Could you check a few things on this model? Use its own coordinates, in mm. A direction names the side the tool comes from. Coordinates: 2 decimals unless noted, no trailing zeros. Loops run counter-clockwise (first coordinate to the right, second up) from the corner with the lowest first, then second, coordinate; pieces in that order, holes last.
from build123d import *

# Parameters (mm, degrees)
SKETCH_R        = 6
SKETCH_R_2      = 4
PAD_DEPTH       = 8
PAD001_DEPTH    = 3
SKETCH002_W     = 2
SKETCH002_H     = 10
SKETCH002_W_2   = 10
SKETCH002_H_2   = 2
PAD002_DEPTH    = 2
CHAMFER_SIZE    = 1.99
CHAMFER001_SIZE = 1.99
PAD003_DEPTH    = 6
PAD003_FACE20_W = 5.5
PAD003_FACE20_H = 5.5
POCKET_DEPTH    = 11.001
FILLET_R        = 1
CHAMFER002_SIZE = 1.5


with BuildPart() as part:
    # Sketch → Pad (new body)
    with BuildSketch(Plane.XY):
        with Locations((15, 15)):
            Circle(SKETCH_R)
        with Locations((15, 15)):
            Circle(SKETCH_R_2, mode=Mode.SUBTRACT)
    extrude(amount=PAD_DEPTH)

    # Sketch001 (on Face4 of Pad) → Pad001 (join)
    with BuildSketch(Plane.XY.offset(8)):
        with BuildLine():
            Line((0, 28.183589), (0, 0))
            Line((0, 0), (28.371979, 0))
            ThreePointArc((28.371979, 0), (29.515053, 0.439592), (29.949498, 1.584632))
            ThreePointArc((29.949498, 1.584632), (21.158025, 21.174653), (1.561155, 29.950849))
            ThreePointArc((1.561155, 29.950849), (0.351368, 29.446372), (0, 28.183589))
        make_face()
    extrude(amount=PAD001_DEPTH)

    # Sketch002 (on Face4 of Pad001) → Pad002 (join)
    with BuildSketch(Plane(origin=(0, 0, 8), x_dir=(1, 0, 0), z_dir=(0, 0, -1))):
        with Locations((6, -15)):
            Rectangle(SKETCH002_W, SKETCH002_H)
        with Locations((15, -6)):
            Rectangle(SKETCH002_W_2, SKETCH002_H_2)
    extrude(amount=PAD002_DEPTH)

    # Chamfer
    chamfer_edges = [part.edges().sort_by_distance(p)[0] for p in [
        (11, 15, 8),
    ]]
    chamfer(chamfer_edges, length=CHAMFER_SIZE)

    # Chamfer001
    chamfer001_edges = [part.edges().sort_by_distance(p)[0] for p in [
        (5, 15, 8),
        (15, 5, 8),
    ]]
    chamfer(chamfer001_edges, length=CHAMFER001_SIZE)

    # Sketch003 → Pad003 (join)
    with BuildSketch(Plane.XY.offset(11)):
        Polygon((0, 8.5), (8.5, 8.5), (8.5, 0), (5.5, 0), (5.5, 5.5), (0, 5.5), align=None)
    extrude(amount=PAD003_DEPTH)

    # Pad003 Face20 → Pocket (cut, through all)
    with BuildSketch(Plane(origin=(2.75, 2.75, 11), x_dir=(0, 1, 0), z_dir=(0, 0, 1))):
        Rectangle(PAD003_FACE20_W, PAD003_FACE20_H)
    extrude(amount=-POCKET_DEPTH, mode=Mode.SUBTRACT)

    # Fillet
    fillet_edges = [part.edges().sort_by_distance(p)[0] for p in [
        (29.515053, 0.439592, 11),
        (18.435989, 0, 11),
        (21.158025, 21.174653, 11),
        (0.351368, 29.446372, 11),
        (0, 18.341794, 11),
    ]]
    fillet(fillet_edges, radius=FILLET_R)

    # Chamfer002
    chamfer002_edges = [part.edges().sort_by_distance(p)[0] for p in [
        (2.75, 5.5, 17),
        (5.5, 2.75, 17),
    ]]
    chamfer(chamfer002_edges, length=CHAMFER002_SIZE)


solid = part.part
1) If I drill on L1, parallel to Y at x = 15, z = 4.25; L2, parallel to Z at x = 2, y = 18.5; L3, parallel to Y at x = 3.5, z = 11.5, over which ranges is the centre line in solid material (lowest first)?
2) For faces 1 (the cylindrical face through (20.54, 12.7, 3.94)), 2 (the flat face through (5.5, 3, 12)), 3 (the flat face through (15, 6, 6)), which set-ups out of +Z, -Z, +X, -X, +Y, -Y let a thin tool reach every point of the face, with its end or its side?
3) Imagine slicing it at A-A on z = 13.5. List the corners of the cut face in (x, y) for me, plus the area to 3 significant figures.
4) Will these pins go through, and if not, where does the flat tip stop? pin 1 (2 mm diameter, centred on y = 4, z = 15, fed in from +X); pin 2 (8 mm diameter, centred on x = 10.5, y = 10, fed in from -Z); pin 3 (6 mm diameter, centred on x = 25.5, z = 13, fed in from +Y); pin 4 (8 mm diameter, centred on x = 10, z = 2, fed in from +Y).
5) We'd pull the mould along Y, two halves only. Please class faces 4 (the cylindrical face through (12.05, 17.7, 2.96)), 5 (the flat face through (4.02, 15.07, 6.99)), 6 (the flat face through (5, 10, 7)), 7 (the cylindrical face through (21.37, 20.96, 8.99)): released by +Y, released by -Y, zero draft, split by the parting line, or undercut.
Solved:
1. L1: y = 9 to 11, 19 to 21
1. L2: z = 8 to 11
1. L3: y = 5.5 to 8.5
2. face 1: -Z
2. face 2: +Z, -Z, -X, -Y
2. face 3: -Z, +X, -X, -Y
3. outline: (0, 5.5) - (5.5, 5.5) - (5.5, 0) - (8.5, 0) - (8.5, 8.5) - (0, 8.5) - close
3. area: 42.0 mm2
4. pin 1: stops at x = 8.5
4. pin 2: stops at z = 0
4. pin 3: stops at y = 17.98
4. pin 4: stops at y = 20.92
5. face 4: undercut
5. face 5: zero draft
5. face 6: released by -Y
5. face 7: released by +Y
